Design review of the part built by this model. Coordinates are the model's own, in mm. A direction names the side the tool comes from. Coordinates: 2 decimals unless noted, no trailing zeros. Loops run counter-clockwise (first coordinate to the right, second up) from the corner with the lowest first, then second, coordinate; pieces in that order, holes last. Notation, with made-up numbers: M -32.75,-9.5 L -16.75,-9.5 A21 ccw -16.75,17.5 Z; hole C 14,75 d7. An arc over 180 degrees is marked long. Put each result on its own line as item: value. Start each with the question number.
(1) Take a section at D-D, the plane y = 1.5. Give the boundary of the cut face in (x, z).
(2) The part is to be moulded in two halves that separate along Y. For faces 1 (the flat face through (9, 17, 6)), 2 (the flat face through (5.5, 12, 5)), 3 (the cylindrical face through (34, 19, 2)), say which applies: +Y half, -Y half, draft (parallel to the pull), parting line (faces both ways), or undercut.
(3) For probe 1 along Y at (x, z) = (7.8, 5); probe 2 along X at (y, z) = (17.75, 3.75); probe 3 along X at (y, z) = (10.5, 2), list the stretches that pass through material, from the lowest coordinate up. Write a range as [from, to].
(4) For faces 4 (the cylindrical face through (21, 2, 9)), 5 (the flat face through (31.6, 10.7, 5.1)), 6 (the cylindrical face through (9.5, 19, 4.9)), 7 (the flat face through (36.1, 12, 5)), 8 (the cylindrical face through (21, 1, 2)), list the 3-axis set-ups (+Z, -Z, +X, -X, +Y, -Y) from which the entire face can be reached by the end or side of a thin tool; tool diameter is ignored.
(5) Take a section at B-B, the plane y = 10.25. Give the boundary of the cut face in (x, z).
(6) Clearance check with flat-ended pins moving along their axes: pin 1 (1.6 mm diameter, centred on x = 45, z = 5, fed in from +Y); pin 2 (3 mm diameter, centred on y = 16.5, z = 3, fed in from -X); pin 3 (5 mm diameter, centred on y = 11.5, z = 7, fed in from +X); pin 4 (6 mm diameter, centred on x = -1, y = 10.5, fed in from +Z). State where each tip first meets the part, or that it passes through.
Autodesk Inventor part; units mm, degrees
ref_plane "YZ Plane" through (0, 0, 0) normal (1, 0, 0) x (0, 1, 0)
ref_plane "XZ Plane" through (0, 0, 0) normal (0, 1, 0) x (-1, 0, 0)
ref_plane "XY Plane" through (0, 0, 0) normal (0, 0, 1) x (1, 0, 0)
sketch "Sketch1" plane through (0, 0, 0) normal (0, 0, 1) x (1, 0, 0)
  line L0 (0, 0) -> (41.6, 0)
  line L1 (41.6, 0) -> (41.6, 20)
  line L2 (41.6, 20) -> (0, 20)
  line L3 (0, 20) -> (0, 0)
  dimension "d0" = 41.6
  dimension "d1" = 20
extrude "Extrusion1" add sketch "Sketch1" along normal blind 10
sketch "Sketch3" plane through (0, 0, 10) normal (0, 0, 1) x (1, 0, 0)
  line L0 (0, 20) -> (5, 20)
  line L1 (5, 20) -> (5, 10)
  line L2 (5, 10) -> (0, 10)
  line L3 (0, 10) -> (0, 20)
  line L4 (41.6, 20) -> (36.6, 20)
  line L5 (36.6, 20) -> (36.6, 10)
  line L6 (36.6, 10) -> (41.6, 10)
  line L7 (41.6, 10) -> (41.6, 20)
  dimension "d7" = 5
  dimension "d8" = 5
  dimension "d9" = 10
extrude "Extrusion2" cut sketch "Sketch3" against normal through all
sketch "Sketch4" plane through (0, 0, 10) normal (0, 0, 1) x (1, 0, 0)
  line L0 (36.6, 20) -> (5, 20)
  line L1 (5, 20) -> (5, 10)
  line L2 (10, 20) -> (31.6, 20)
  line L3 (31.6, 20) -> (31.6, 10)
  line L4 (31.6, 10) -> (10, 10)
  line L5 (10, 10) -> (10, 20)
  dimension "d12" = 21.6
  dimension "d13" = 10
  dimension "d14" = 5
extrude "Extrusion3" cut sketch "Sketch4" against normal through all
fillet "Fillet1" radius 5 6 edges at (20.8, 0, 0) (20.8, 0, 10) (34.1, 20, 10) (34.1, 20, 0) (7.5, 20, 0) (7.5, 20, 10)
sketch "Sketch5" plane through (10, 10, 10) normal (0, 1, 0) x (1, 0, 0)
  line L0 (0, 10) -> (21.6, 10)
  line L1 (0, 0) -> (0, 10)
  line L2 (21.6, 0) -> (0, 0)
  line L3 (21.6, 0) -> (21.6, 10)
  point P0 (-10, 10)
extrude "Extrusion4" cut sketch "Sketch5" against normal blind 5
sketch "Sketch6" plane through (36.6, 10, 10) normal (0, 1, 0) x (1, 0, 0)
  line L0 (0, 10) -> (5, 10)
  line L1 (0, 0) -> (0, 10)
  line L2 (5, 0) -> (0, 0)
  line L3 (5, 10) -> (5, 0)
  point P0 (-36.6, 10)
extrude "Extrusion5" cut sketch "Sketch6" against normal blind 5
sketch "Sketch7" plane through (0, 10, 10) normal (0, 1, 0) x (1, 0, 0)
  line L0 (0, 10) -> (5, 10)
  line L1 (0, 0) -> (0, 10)
  line L2 (5, 0) -> (0, 0)
  line L3 (5, 0) -> (5, 10)
extrude "Extrusion6" cut sketch "Sketch7" against normal blind 5
sketch "Sketch8" plane through (5, 15, 5) normal (-1, 0, 0) x (0, 0, 1)
  arc A0 (5, 0) -> (-5, 0) centre (0, 0) ccw
  line L0 (-5, -10) -> (-5, 0)
  line L1 (-5, -10) -> (5, -10)
  line L2 (5, 0) -> (5, -10)
  point P0 (-5, -15)
extrude "Extrusion7" cut sketch "Sketch8" against normal blind 0.5
sketch "Sketch9" plane through (36.6, 15, 5) normal (1, 0, 0) x (0, 0, -1)
  arc A0 (5, 0) -> (-5, 0) centre (0, 0) ccw
  line L0 (-5, -10) -> (-5, 0)
  line L1 (-5, -10) -> (5, -10)
  line L2 (5, 0) -> (5, -10)
  point P0 (5, -15)
extrude "Extrusion8" cut sketch "Sketch9" against normal blind 0.5
sketch "Sketch10" plane through (36.1, 15, 5) normal (1, 0, 0) x (0, 0, -1)
  arc A0 (5, 0) -> (-5, 0) centre (0, 0) ccw
  circle A1 centre (0, 0) radius 2
  point P0 (5, -15)
  dimension "d28" = 4
extrude "Extrusion9" cut sketch "Sketch10" against normal through all
sketch "Sketch11" plane through (31.6, 15, 5) normal (-1, 0, 0) x (0, 0, 1)
  circle A0 centre (0, 0) radius 2
  arc A1 (5, 0) -> (-5, 0) centre (0, 0) ccw
  line L0 (5, 0) -> (5, -10)
  line L1 (-3.7, 1.5199) -> (-3.7, -1.5199)
  line L2 (3.7, 1.5199) -> (3.7, -1.5199)
  arc A2 (-3.7, -1.5199) -> (3.7, -1.5199) centre (0, 0) ccw
  arc A3 (3.7, 1.5199) -> (-3.7, 1.5199) centre (0, 0) ccw
  point P0 (-5, -15)
  dimension "d33" = 3.7
extrude "Extrusion10" cut sketch "Sketch11" against normal blind 1
sketch "Sketch12" plane through (10, 15, 5) normal (1, 0, 0) x (0, 0, -1)
  circle A0 centre (0, 0) radius 2
  arc A1 (5, 0) -> (-5, 0) centre (0, 0) ccw
  line L0 (5, 0) -> (5, -10)
  line L1 (3.7, 1.5199) -> (3.7, -1.5199)
  line L2 (-3.7, 1.5199) -> (-3.7, -1.5199)
  arc A2 (-3.7, -1.5199) -> (3.7, -1.5199) centre (0, 0) ccw
  arc A3 (3.7, 1.5199) -> (-3.7, 1.5199) centre (0, 0) ccw
  point P0 (5, -15)
  dimension "d37" = 3.7
extrude "Extrusion11" cut sketch "Sketch12" against normal blind 1
sketch "Sketch13" plane through (41.6, 5, 5) normal (1, 0, 0) x (0, 0, -1)
  line L0 (5, 0) -> (-5, 0)
  arc A0 (-5, 0) -> (5, 0) centre (0, 0) ccw
  point P0 (5, -5)
extrude "Extrusion12" add sketch "Sketch13" along normal blind 1
sketch "Sketch14" plane through (0, 5, 5) normal (-1, 0, 0) x (0, 0, 1)
  line L0 (5, 0) -> (-5, 0)
  arc A0 (-5, 0) -> (5, 0) centre (0, 0) ccw
  point P0 (-5, -5)
extrude "Extrusion13" add sketch "Sketch14" along normal blind 1
sketch "Sketch15" plane through (36.6, 5, 10) normal (0, 1, 0) x (1, 0, 0)
  line L0 (-0.5, 10) -> (6, 10)
  line L1 (-0.5, 10) -> (-0.5, 0)
  line L2 (-0.5, 0) -> (6, 0)
  line L3 (6, 10) -> (6, 0)
  point P0 (-36.6, 10)
extrude "Extrusion14" add sketch "Sketch15" along normal blind 2
sketch "Sketch16" plane through (10, 5, 10) normal (0, 1, 0) x (1, 0, 0)
  line L0 (0, 10) -> (21.6, 10)
  line L1 (0, 0) -> (0, 10)
  line L2 (21.6, 0) -> (0, 0)
  line L3 (21.6, 10) -> (21.6, 0)
  point P0 (-10, 10)
extrude "Extrusion15" add sketch "Sketch16" along normal blind 2
sketch "Sketch17" plane through (0, 5, 10) normal (0, 1, 0) x (1, 0, 0)
  line L0 (-1, 10) -> (5.5, 10)
  line L1 (-1, 0) -> (-1, 10)
  line L2 (5.5, 0) -> (-1, 0)
  line L3 (5.5, 0) -> (5.5, 10)
  point P0 (0, 10)
extrude "Extrusion16" add sketch "Sketch17" along normal blind 2
sketch "Sketch18" plane through (-1, 5, 5) normal (-1, 0, 0) x (0, 0, 1)
  arc A0 (-5, 0) -> (5, 0) centre (0, 0) ccw
  line L0 (5, 0) -> (5, 2)
  line L1 (-5, 2) -> (5, 2)
  line L2 (-5, 0) -> (-5, 2)
  point P0 (-5, -5)
extrude "Extrusion17" add sketch "Sketch18" along normal blind 5.4
sketch "Sketch19" plane through (42.6, 5, 5) normal (1, 0, 0) x (0, 0, -1)
  arc A0 (-5, 0) -> (5, 0) centre (0, 0) ccw
  line L0 (5, 0) -> (5, 2)
  line L1 (-5, 2) -> (5, 2)
  line L2 (-5, 0) -> (-5, 2)
  point P0 (5, -5)
extrude "Extrusion18" add sketch "Sketch19" along normal blind 5.4
properties part number "Slide"
Computed values:
1. outline: M -6.4,1.43 L 0,1.43 L 41.6,1.43 L 48,1.43 L 48,8.57 L 41.6,8.57 L 0,8.57 L -6.4,8.57 Z
2. face 1: undercut
2. face 2: draft
2. face 3: +Y half
3. probe 1: y = [0, 13], [17, 20]
3. probe 2: x = [5.5, 9], [32.6, 36.1]
3. probe 3: x = [5.5, 10], [31.6, 36.1]
4. face 4: +Z, +X, -X, -Y
4. face 5: +Z, -Z, +Y
4. face 6: none
4. face 7: +Z, -Z, +X, +Y
4. face 8: -Z, +X, -X, -Y
5. outline: M 5.5,0 L 10,0 L 10,10 L 5.5,10 Z; M 31.6,0 L 36.1,0 L 36.1,10 L 31.6,10 Z
6. pin 1: stops at y = 7
6. pin 2: stops at x = 5.5
6. pin 3: stops at x = 36.1
6. pin 4: passes through
